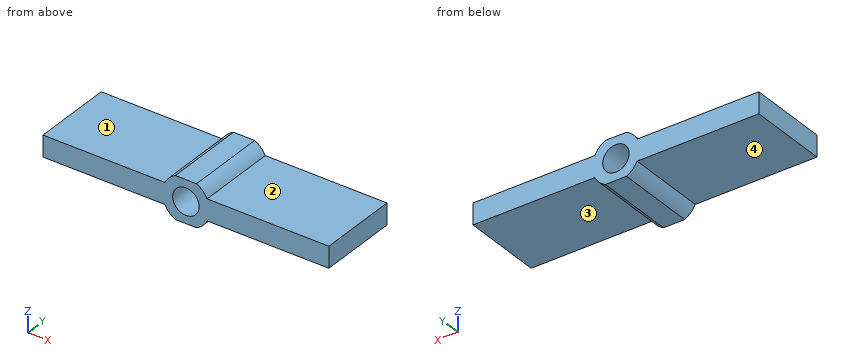
```python
from build123d import *

# Parameters (mm, degrees)
SKETCH1_W                = 11.5
SKETCH1_H                = 7.6
BOSS_EXTRUDE5_DEPTH      = 1
BOSS_EXTRUDE5_2_DEPTH    = 1
SKETCH1_5_W              = 11.5
SKETCH1_5_H              = 7.6
BOSS_EXTRUDE6_DEPTH      = 1
BOSS_EXTRUDE7_DEPTH      = 2
BOSS_EXTRUDE7_DEPTH_BACK = 2
SKETCH1_6_W              = 4
SKETCH1_6_H              = 7.6
SKETCH2_R                = 1.25
CUT_EXTRUDE1_DEPTH       = 9


with BuildPart() as part:
    # Sketch1 → Boss-Extrude5 (new body)
    with BuildSketch(Plane.XY):
        with Locations((5.75, 3.8)):
            Rectangle(SKETCH1_W, SKETCH1_H)
    extrude(amount=BOSS_EXTRUDE5_DEPTH)



with BuildPart() as body_2:
    # Sketch1 → Boss-Extrude5 2 (new body)
    with BuildSketch(Plane.XY):
        with Locations((21.25, 3.8)):
            Rectangle(SKETCH1_W, SKETCH1_H)
    extrude(amount=BOSS_EXTRUDE5_2_DEPTH)


with BuildPart() as part_1:
    add(part.part)

    add(body_2.part)  # Boss-Extrude6 merges body 2
    # Sketch1_5 → Boss-Extrude6 (add)
    with BuildSketch(Plane.XY):
        with Locations((21.25, 3.8)):
            Rectangle(SKETCH1_5_W, SKETCH1_5_H)
        with Locations((5.75, 3.8)):
            Rectangle(SKETCH1_5_W, SKETCH1_5_H)
    extrude(amount=-BOSS_EXTRUDE6_DEPTH)

    # Sketch1_6 → Boss-Extrude7 (add, two sides: drawn at the far end of the back side and taken through both)
    with BuildSketch(Plane.XY.offset(-BOSS_EXTRUDE7_DEPTH_BACK)):
        with Locations((13.5, 3.8)):
            Rectangle(SKETCH1_6_W, SKETCH1_6_H)
    extrude(amount=BOSS_EXTRUDE7_DEPTH + BOSS_EXTRUDE7_DEPTH_BACK)

    # Sketch2 → Cut-Extrude1 (cut)
    with BuildSketch(Plane(origin=(0, 7.6, 0), x_dir=(1, 0, 0), z_dir=(0, 1, 0))):
        with BuildLine():
            Line((12.5, 2), (11.5, 2))
            Line((11.5, 2), (11.5, 1))
            ThreePointArc((11.5, 1), (11.91886117, 1.58113883), (12.5, 2))
        make_face()
        with BuildLine():
            Line((15.5, 2), (14.5, 2))
            ThreePointArc((14.5, 2), (15.08113883, 1.58113883), (15.5, 1))
            Line((15.5, 1), (15.5, 2))
        make_face()
        with BuildLine():
            Line((15.5, -2), (15.5, -1))
            ThreePointArc((15.5, -1), (15.08113883, -1.58113883), (14.5, -2))
            Line((14.5, -2), (15.5, -2))
        make_face()
        with BuildLine():
            ThreePointArc((12.5, -2), (11.91886117, -1.58113883), (11.5, -1))
            Line((11.5, -1), (11.5, -2))
            Line((11.5, -2), (12.5, -2))
        make_face()
        with Locations(Location((13.5, 0, 0), (0, 0, 270))):
            Circle(SKETCH2_R)
    extrude(amount=-CUT_EXTRUDE1_DEPTH, mode=Mode.SUBTRACT)


solid = part_1.part
```
Source: CAD feature listing. Evaluate the final solid. Frame: model axes, mm. Face numbers are marked on the shaded views. A direction names the side the tool comes from. Round coordinates to 2 decimals unless told otherwise and drop trailing zeros. Loops run counter-clockwise (first coordinate to the right, second up) from the corner with the lowest first, then second, coordinate; pieces in that order, holes last.
1. Contact query for flat-ended pins moving along their axis: pin 1 (1 mm diameter, centred on x = 6, y = 6, fed in from +Z); pin 2 (4 mm diameter, centred on x = 8.5, y = 4.5, fed in from -Z). Output: stop coordinate, or through.
2. Ray query, L1, parallel to X at y = 3.25, z = 0; L2, parallel to Z at x = 17.25, y = 3; L3, parallel to Z at x = 13, y = 4. Return the intervals inside material, ascending.
3. Section query A-A on z = 0. Output: boundary loops of the cut face in (x, y).
4. Section query D-D on z = 1.65. Output: boundary loops of the cut face in (x, y), and give its area (3 significant figures).
5. Section query B-B on y = 4.5. Output: boundary loops of the cut face in (x, z), and give its area (3 significant figures).
6. Section query C-C on x = 5.5. Output: boundary loops of the cut face in (y, z), and give its area (3 significant figures).
7. Access query for the marked faces 1, 2, 3 and 4. Directions: +Z, -Z, +X, -X, +Y, -Y. A direction counts if a zero-diameter tool reaches every point of the face in a straight line with its end or side. Return the directions, or none.
Answers below:
1. pin 1: stops at z = 1
1. pin 2: stops at z = -1
2. L1: x = 0 to 12.25, 14.75 to 27
2. L2: z = -1 to 1
2. L3: z = -2 to -1.15, 1.15 to 2
3. outline: (0, 0) - (12.25, 0) - (12.25, 7.6) - (0, 7.6) - close; (14.75, 0) - (27, 0) - (27, 7.6) - (14.75, 7.6) - close
4. outline: (11.99, 0) - (15.01, 0) - (15.01, 7.6) - (11.99, 7.6) - close
4. area: 22.9 mm2
5. outline: (0, -1) - (11.5, -1) arc R2.24 ccw to (12.5, -2) - (14.5, -2) arc R2.24 ccw to (15.5, -1) - (27, -1) - (27, 1) - (15.5, 1) arc R2.24 ccw to (14.5, 2) - (12.5, 2) arc R2.24 ccw to (11.5, 1) - (0, 1) - close; hole circle Ø2.5 at (13.5, 0)
5. area: 55.5 mm2
6. outline: (0, -1) - (7.6, -1) - (7.6, 1) - (0, 1) - close
6. area: 15.2 mm2
7. face 1: +Z, -X, +Y, -Y
7. face 2: +Z, +X, +Y, -Y
7. face 3: -Z, +X, +Y, -Y
7. face 4: -Z, -X, +Y, -Y
